```python
from build123d import *

# Parameters (mm, degrees)
ESQUISSE1_W             = 61
ESQUISSE1_H             = 78
BOSS_EXTRU_1_DEPTH      = 2
ESQUISSE2_W             = 61
ESQUISSE2_H             = 78
ESQUISSE2_W_2           = 57
ESQUISSE2_H_2           = 74
BOSS_EXTRU_2_DEPTH      = 12
ESQUISSE3_W             = 61
ESQUISSE3_H             = 78
ESQUISSE3_W_2           = 59
ESQUISSE3_H_2           = 76
BOSS_EXTRU_3_DEPTH      = 4
ESQUISSE7_W             = 17
ESQUISSE7_H             = 20.984875374
ESQUISSE7_W_2           = 7
ESQUISSE7_H_2           = 18.09159362
ESQUISSE7_W_3           = 9.5
ESQUISSE7_H_3           = 11.016430182
ENL_V_MAT_EXTRU_2_DEPTH = 3
ENL_V_MAT_EXTRU_3_REACH = 54.681
ESQUISSE8_W             = 4
ESQUISSE8_H             = 39
ESQUISSE8_H_2           = 49
ESQUISSE8_W_2           = 11
ESQUISSE8_H_3           = 6
CHANFREIN1_SIZE         = 2
ENL_V_MAT_EXTRU_4_REACH = 54.681
ESQUISSE9_R             = 2.5
ESQUISSE9_R_2           = 0.75
CONG_1_R                = 1


with BuildPart() as part:
    # Esquisse1 → Boss.-Extru.1 (new body)
    with BuildSketch(Plane.XY):
        Rectangle(ESQUISSE1_W, ESQUISSE1_H)
    extrude(amount=BOSS_EXTRU_1_DEPTH)

    # Esquisse2 → Boss.-Extru.2 (add)
    with BuildSketch(Plane.XY.offset(2)):
        Rectangle(ESQUISSE2_W, ESQUISSE2_H)
        Rectangle(ESQUISSE2_W_2, ESQUISSE2_H_2, mode=Mode.SUBTRACT)
    extrude(amount=BOSS_EXTRU_2_DEPTH)

    # Esquisse3 → Boss.-Extru.3 (add)
    with BuildSketch(Plane.XY.offset(14)):
        Rectangle(ESQUISSE3_W, ESQUISSE3_H)
        Rectangle(ESQUISSE3_W_2, ESQUISSE3_H_2, mode=Mode.SUBTRACT)
    extrude(amount=BOSS_EXTRU_3_DEPTH)

    # Esquisse7 → Enlèv. mat.-Extru.2 (cut)
    with BuildSketch(Plane(origin=(0, 39, 0), x_dir=(1, 0, 0), z_dir=(0, 1, 0))):
        with Locations((-13.5, -14.492437687)):
            Rectangle(ESQUISSE7_W, ESQUISSE7_H)
        with Locations((18, -12.04579681)):
            Rectangle(ESQUISSE7_W_2, ESQUISSE7_H_2)
        with Locations((7.75, -17.508215091)):
            Rectangle(ESQUISSE7_W_3, ESQUISSE7_H_3)
    extrude(amount=-ENL_V_MAT_EXTRU_2_DEPTH, mode=Mode.SUBTRACT)

    # Esquisse8 → Enlèv. mat.-Extru.3 (cut, up to next)
    with BuildSketch(Plane(origin=(0, 0, 0), x_dir=(-1, 0, 0), z_dir=(0, 0, -1)), mode=Mode.PRIVATE) as enl_v_mat_extru_3_sk1:
        with Locations((-24.5, -12.5)):
            Rectangle(ESQUISSE8_W, ESQUISSE8_H)
    enl_v_mat_extru_3_tool1 = extrude(enl_v_mat_extru_3_sk1.sketch, amount=-ENL_V_MAT_EXTRU_3_REACH, mode=Mode.PRIVATE) & part.part
    # Esquisse8 → Enlèv. mat.-Extru.3 (cut, up to next)
    with BuildSketch(Plane(origin=(0, 0, 0), x_dir=(-1, 0, 0), z_dir=(0, 0, -1)), mode=Mode.PRIVATE) as enl_v_mat_extru_3_sk2:
        with Locations((24.5, -7.5)):
            Rectangle(ESQUISSE8_W, ESQUISSE8_H_2)
    enl_v_mat_extru_3_tool2 = extrude(enl_v_mat_extru_3_sk2.sketch, amount=-ENL_V_MAT_EXTRU_3_REACH, mode=Mode.PRIVATE) & part.part
    # Esquisse8 → Enlèv. mat.-Extru.3 (cut, up to next)
    with BuildSketch(Plane(origin=(0, 0, 0), x_dir=(-1, 0, 0), z_dir=(0, 0, -1)), mode=Mode.PRIVATE) as enl_v_mat_extru_3_sk3:
        with Locations((-11, -32)):
            Rectangle(ESQUISSE8_W_2, ESQUISSE8_H_3)
    enl_v_mat_extru_3_tool3 = extrude(enl_v_mat_extru_3_sk3.sketch, amount=-ENL_V_MAT_EXTRU_3_REACH, mode=Mode.PRIVATE) & part.part
    add(enl_v_mat_extru_3_tool1.solids().sort_by_distance((24.5, -12.5, 0))[0], mode=Mode.SUBTRACT)
    add(enl_v_mat_extru_3_tool2.solids().sort_by_distance((-24.5, -7.5, 0))[0], mode=Mode.SUBTRACT)
    add(enl_v_mat_extru_3_tool3.solids().sort_by_distance((11, -32, 0))[0], mode=Mode.SUBTRACT)

    # Chanfrein1
    chanfrein1_edges = [part.edges().sort_by_distance(p)[0] for p in [
        (-28.5, -37, 8),
        (28.5, -37, 8),
        (28.5, 37, 8),
        (-28.5, 37, 8),
    ]]
    chamfer(chanfrein1_edges, length=CHANFREIN1_SIZE)

    # Esquisse9 → Enlèv. mat.-Extru.4 (cut, up to next)
    with BuildSketch(Plane(origin=(0, 0, 0), x_dir=(-1, 0, 0), z_dir=(0, 0, -1)), mode=Mode.PRIVATE) as enl_v_mat_extru_4_sk1:
        with Locations((0, -9)):
            Circle(ESQUISSE9_R)
    enl_v_mat_extru_4_tool1 = extrude(enl_v_mat_extru_4_sk1.sketch, amount=-ENL_V_MAT_EXTRU_4_REACH, mode=Mode.PRIVATE) & part.part
    # Esquisse9 → Enlèv. mat.-Extru.4 (cut, up to next)
    with BuildSketch(Plane(origin=(0, 0, 0), x_dir=(-1, 0, 0), z_dir=(0, 0, -1)), mode=Mode.PRIVATE) as enl_v_mat_extru_4_sk2:
        with Locations((-7, -9)):
            Circle(ESQUISSE9_R_2)
    enl_v_mat_extru_4_tool2 = extrude(enl_v_mat_extru_4_sk2.sketch, amount=-ENL_V_MAT_EXTRU_4_REACH, mode=Mode.PRIVATE) & part.part
    # Esquisse9 → Enlèv. mat.-Extru.4 (cut, up to next)
    with BuildSketch(Plane(origin=(0, 0, 0), x_dir=(-1, 0, 0), z_dir=(0, 0, -1)), mode=Mode.PRIVATE) as enl_v_mat_extru_4_sk3:
        with Locations((7, -9)):
            Circle(ESQUISSE9_R_2)
    enl_v_mat_extru_4_tool3 = extrude(enl_v_mat_extru_4_sk3.sketch, amount=-ENL_V_MAT_EXTRU_4_REACH, mode=Mode.PRIVATE) & part.part
    # Esquisse9 → Enlèv. mat.-Extru.4 (cut, up to next)
    with BuildSketch(Plane(origin=(0, 0, 0), x_dir=(-1, 0, 0), z_dir=(0, 0, -1)), mode=Mode.PRIVATE) as enl_v_mat_extru_4_sk4:
        with Locations((0, -2)):
            Circle(ESQUISSE9_R_2)
    enl_v_mat_extru_4_tool4 = extrude(enl_v_mat_extru_4_sk4.sketch, amount=-ENL_V_MAT_EXTRU_4_REACH, mode=Mode.PRIVATE) & part.part
    # Esquisse9 → Enlèv. mat.-Extru.4 (cut, up to next)
    with BuildSketch(Plane(origin=(0, 0, 0), x_dir=(-1, 0, 0), z_dir=(0, 0, -1)), mode=Mode.PRIVATE) as enl_v_mat_extru_4_sk5:
        with Locations((0, -16)):
            Circle(ESQUISSE9_R_2)
    enl_v_mat_extru_4_tool5 = extrude(enl_v_mat_extru_4_sk5.sketch, amount=-ENL_V_MAT_EXTRU_4_REACH, mode=Mode.PRIVATE) & part.part
    add(enl_v_mat_extru_4_tool1.solids().sort_by_distance((0, -9, 0))[0], mode=Mode.SUBTRACT)
    add(enl_v_mat_extru_4_tool2.solids().sort_by_distance((7, -9, 0))[0], mode=Mode.SUBTRACT)
    add(enl_v_mat_extru_4_tool3.solids().sort_by_distance((-7, -9, 0))[0], mode=Mode.SUBTRACT)
    add(enl_v_mat_extru_4_tool4.solids().sort_by_distance((0, -2, 0))[0], mode=Mode.SUBTRACT)
    add(enl_v_mat_extru_4_tool5.solids().sort_by_distance((0, -16, 0))[0], mode=Mode.SUBTRACT)

    # Congé1
    cong_1_edges = [part.edges().sort_by_distance(p)[0] for p in [
        (0, 37, 2),
        (-28.5, 0, 2),
        (0, -37, 2),
        (28.5, 0, 2),
        (27.5, 36, 2),
        (27.5, -36, 2),
        (-27.5, -36, 2),
        (-27.5, 36, 2),
    ]]
    fillet(cong_1_edges, radius=CONG_1_R - 0.0001)  # a hair under: the kernel refuses the full size


solid = part.part
```
Verification items for the finished model (mm, model axes). A direction names the side the tool comes from. Coordinates: 2 decimals unless noted, no trailing zeros. Write each loop counter-clockwise with the first axis right and the second up, starting at its lowest first coordinate (ties: lowest second). Pieces come first, ordered by that corner, then holes. Notation, with made-up numbers: (83.5, -9.5) - (122.5, -9.5) arc R6 cw to (122.5, -2.5) - close; hole circle Ø2 at (84, 76). An arc over 180 degrees is marked (long way). One line per question, with ' | ' between items. Start each with the question number.
1. Access from +Z, -Z, +X, -X, +Y, -Y to the whole of each face (thin tool, end or side, straight path). Record for faces 1 (the flat face through (26.5, -13, 1)), 2 (the flat face through (8, 38, 12)), 3 (the flat face through (25, 38, 16)).
2. Section check C-C (y = 19). Enter the section's corners in (x, z), plus the area to 3 significant figures.
3. Draft check along X on faces 4 (the flat face through (0, 1, 0)), 5 (the flat face through (-30.5, -1, 9)), 6 (the flat face through (-29.5, -1, 16)). Enter one of: released by +X, released by -X, zero draft, split by the parting line, or undercut.
4. Section check A-A (x = -17.5). Enter the section's corners in (y, z), plus the area to 3 significant figures.
5. Gauge pin test, flat ends, axial feed: P1, Ø0.9, axis at x = 0, y = -2, coming from the +Z side; P2, Ø5, axis at x = -8.5, y = 0, coming from the +Z side; P3, Ø1.6, axis at x = 19, y = 37.5, coming from the +Z side. Record the tip position at first contact, or that the pin passes through.
6. Section check B-B (y = -19). Enter the section's corners in (x, z).
7. Material ranges on line 1 along Y through (x, z) = (7, 1.15); line 2 along X through (y, z) = (-28, 1.25); line 3 along Y through (x, z) = (-3, 12.25), recorded low to high.
Computed values:
1) face 1: +Z, -Z | face 2: +Z, +Y | face 3: +Z
2) outline: (-30.5, 0) - (30.5, 0) - (30.5, 18) - (29.5, 18) - (29.5, 14) - (28.5, 14) - (28.5, 3) arc R1 cw to (27.5, 2) - (-27.5, 2) arc R1 cw to (-28.5, 3) - (-28.5, 14) - (-29.5, 14) - (-29.5, 18) - (-30.5, 18) - close | area: 178 mm²
3) face 4: zero draft | face 5: released by -X | face 6: undercut
4) outline: (-39, 0) - (39, 0) - (39, 4) - (37, 4) - (37, 3) arc R1 cw to (36, 2) - (-36, 2) arc R1 cw to (-37, 3) - (-37, 14) - (-38, 14) - (-38, 18) - (-39, 18) - close | area: 188 mm²
5) P1: through | P2: z = 2 | P3: z = 3
6) outline: (-30.5, 0) - (-26.5, 0) - (-26.5, 2) - (-27.5, 2) arc R1 cw to (-28.5, 3) - (-28.5, 14) - (-29.5, 14) - (-29.5, 18) - (-30.5, 18) - close; (-22.5, 0) - (22.5, 0) - (22.5, 2) - (-22.5, 2) - close; (26.5, 0) - (30.5, 0) - (30.5, 18) - (29.5, 18) - (29.5, 14) - (28.5, 14) - (28.5, 3) arc R1 cw to (27.5, 2) - (26.5, 2) - close
7) line 1: -39 to -35, -29 to -9.75, -8.25 to 39 | line 2: -30.5 to -26.5, -22.5 to 22.5, 26.5 to 30.5 | line 3: -39 to -37, 37 to 39
